Geometry check sheet. Reference: drawing and pictorial views, mm from the part's lowest x, y, z. A direction names the side the tool comes from. Give positions to 0.01 mm unless a question says otherwise; leave off trailing zeros. Answer as a JSON object with one key per item and string values.
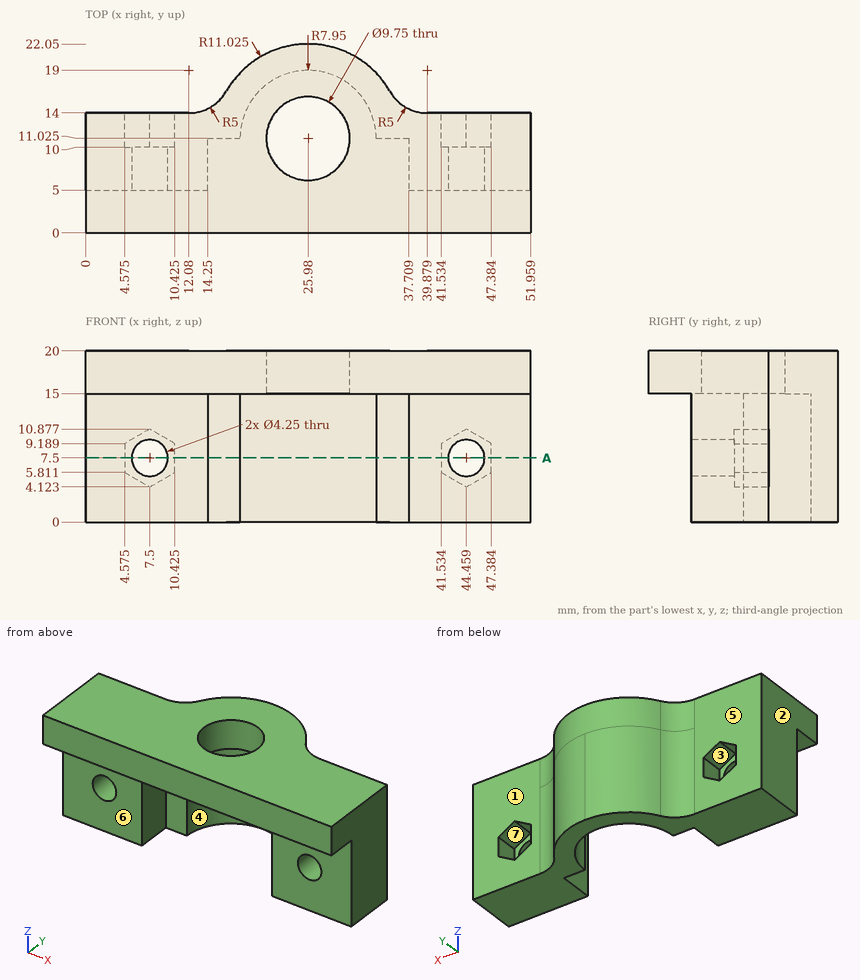
1) Thickness scan on L1, parallel to Y at x = 11.5, z = 4.5; L2, parallel to X at y = 13.5, z = 15.5; L3, parallel to Y at x = 7, z = 15.5. Record the ranges inside material, lowest first.
Completed:
{"L1": "y = 5 to 14", "L2": "x = 0 to 21.78, 30.18 to 51.96", "L3": "y = 0 to 14"}
2) Go/stop test with flat-tipped pins: pin 1 (4.5 mm diameter, centred on x = 8.5, z = 7.5, fed in from +Y); pin 2 (1.1 mm diameter, centred on x = 36, z = 10.5, fed in from -Y) (1 decimal); pin 3 (8 mm diameter, centred on x = 39.5, z = 9.5, fed in from +Y) (1 decimal). Record where each tip stops, or that it passes through.
Completed:
{"pin 1": "stops at y = 14", "pin 2": "stops at y = 11", "pin 3": "stops at y = 16.6"}
3) Release check for a two-part mould opening along X. For the marked faces 1, 2 and 3 record: pulls with the +X half, pulls with the -X half, needs draft (parallel to the pull), parting line crosses it, or undercut.
Completed:
{"face 1": "needs draft", "face 2": "pulls with the -X half", "face 3": "undercut"}
4) Access from +Z, -Z, +X, -X, +Y, -Y to the whole of each face (thin tool, end or side, straight path). Record for the marked faces 4, 5, 6 and 7.
Completed:
{"face 4": "-Z, -Y", "face 5": "+Z, -Z, -X, +Y", "face 6": "-Z, +X, -X, -Y", "face 7": "+Y"}
5) Section check A-A on z = 7.5. Count the separate pieces of the cut face and the enclosed holes in it, and give its area (3 significant figures).
Completed:
{"separate pieces": "3", "enclosed holes": "0", "area": "267 mm2"}
